Check sheet for the modelled part. Datum: model origin and axes. Units: mm. Face numbers are marked on the shaded views. A direction names the side the tool comes from. Round coordinates to 2 decimals unless told otherwise and drop trailing zeros. Order: outer loops, then holes, each group sorted by start corner. A loop starts at its lowest first (then second) coordinate and runs counter-clockwise, first axis right, second up. Notation, with made-up numbers: (-13, 39.5) -> (25, 39.5) arc R35 ccw to (25, 78.5) -> close; hole circle Ø3 at (-9.5, 52.25). An arc over 180 degrees is marked (long way). Answer as CSV lines item,"result". Start each with the question number.
from build123d import *

# Parameters (mm, degrees)
SKETCH1_W      = 16
SKETCH1_H      = 16
EXTRUDE1_DEPTH = 80
SKETCH2_W      = 13
SKETCH2_H      = 13
EXTRUDE2_DEPTH = 84.138438763
SKETCH3_R      = 4
SKETCH3_R_2    = 1.85
EXTRUDE3_DEPTH = 84.138438763
SKETCH4_R      = 4
SKETCH4_R_2    = 1.85
EXTRUDE4_DEPTH = 84.138438763
FILLET1_R      = 1


with BuildPart() as part:
    # Sketch1 → Extrude1 (new body)
    with BuildSketch(Plane.XY):
        with Locations((8, 8)):
            Rectangle(SKETCH1_W, SKETCH1_H)
    extrude(amount=-EXTRUDE1_DEPTH)

    # Sketch2 → Extrude2 (cut, through all)
    with BuildSketch(Plane.XY):
        with Locations((8, 8)):
            Rectangle(SKETCH2_W, SKETCH2_H)
    extrude(amount=-EXTRUDE2_DEPTH, mode=Mode.SUBTRACT)

    # Sketch3 → Extrude3 (cut, through all)
    with BuildSketch(Plane(origin=(0, 16, 0), x_dir=(1, 0, 0), z_dir=(0, 1, 0))):
        with Locations(Location((8, 64, 0), (0, 0, 270))):
            Circle(SKETCH3_R)
        with Locations(Location((8, 32, 0), (0, 0, 270))):
            Circle(SKETCH3_R)
        with Locations((8, 0)):
            Circle(SKETCH3_R)
        with Locations((8, 96)):
            Circle(SKETCH3_R)
        with Locations((8, 128)):
            Circle(SKETCH3_R)
        with Locations((8, 160)):
            Circle(SKETCH3_R)
        with Locations((8, 192)):
            Circle(SKETCH3_R)
        with Locations((8, 224)):
            Circle(SKETCH3_R)
        with Locations((8, 256)):
            Circle(SKETCH3_R)
        with Locations(Location((8, 48, 0), (0, 0, 270))):
            Circle(SKETCH3_R)
        with Locations(Location((8, 56, 0), (0, 0, 270))):
            Circle(SKETCH3_R_2)
        with Locations(Location((8, 40, 0), (0, 0, 270))):
            Circle(SKETCH3_R_2)
        with Locations((8, 80)):
            Circle(SKETCH3_R)
        with Locations((8, 88)):
            Circle(SKETCH3_R_2)
        with Locations(Location((8, 72, 0), (0, 0, 270))):
            Circle(SKETCH3_R_2)
        with Locations(Location((8, 16, 0), (0, 0, 270))):
            Circle(SKETCH3_R)
        with Locations(Location((8, 24, 0), (0, 0, 270))):
            Circle(SKETCH3_R_2)
        with Locations(Location((8, 8, 0), (0, 0, 270))):
            Circle(SKETCH3_R_2)
        with Locations((8, 112)):
            Circle(SKETCH3_R)
        with Locations((8, 120)):
            Circle(SKETCH3_R_2)
        with Locations((8, 104)):
            Circle(SKETCH3_R_2)
        with Locations((8, 144)):
            Circle(SKETCH3_R)
        with Locations((8, 152)):
            Circle(SKETCH3_R_2)
        with Locations((8, 136)):
            Circle(SKETCH3_R_2)
        with Locations((8, 176)):
            Circle(SKETCH3_R)
        with Locations((8, 184)):
            Circle(SKETCH3_R_2)
        with Locations((8, 168)):
            Circle(SKETCH3_R_2)
        with Locations((8, 208)):
            Circle(SKETCH3_R)
        with Locations((8, 216)):
            Circle(SKETCH3_R_2)
        with Locations((8, 200)):
            Circle(SKETCH3_R_2)
        with Locations((8, 240)):
            Circle(SKETCH3_R)
        with Locations((8, 248)):
            Circle(SKETCH3_R_2)
        with Locations((8, 232)):
            Circle(SKETCH3_R_2)
    extrude(amount=-EXTRUDE3_DEPTH, mode=Mode.SUBTRACT)

    # Sketch4 → Extrude4 (cut, through all)
    with BuildSketch(Plane(origin=(16, 0, 0), x_dir=(0, 0, -1), z_dir=(1, 0, 0))):
        with Locations(Location((32, 8, 0), (0, 0, 90))):
            Circle(SKETCH4_R)
        with Locations(Location((64, 8, 0), (0, 0, 90))):
            Circle(SKETCH4_R)
        with Locations((0, 8)):
            Circle(SKETCH4_R)
        with Locations((96, 8)):
            Circle(SKETCH4_R)
        with Locations((128, 8)):
            Circle(SKETCH4_R)
        with Locations((160, 8)):
            Circle(SKETCH4_R)
        with Locations((192, 8)):
            Circle(SKETCH4_R)
        with Locations((224, 8)):
            Circle(SKETCH4_R)
        with Locations((256, 8)):
            Circle(SKETCH4_R)
        with Locations(Location((48, 8.074203, 0), (0, 0, 90))):
            Circle(SKETCH4_R)
        with Locations(Location((40, 8.074203, 0), (0, 0, 90))):
            Circle(SKETCH4_R_2)
        with Locations(Location((56, 8.074203, 0), (0, 0, 90))):
            Circle(SKETCH4_R_2)
        with Locations((80, 8)):
            Circle(SKETCH4_R)
        with Locations(Location((72, 8, 0), (0, 0, 90))):
            Circle(SKETCH4_R_2)
        with Locations((88, 8)):
            Circle(SKETCH4_R_2)
        with Locations(Location((16, 8, 0), (0, 0, 90))):
            Circle(SKETCH4_R)
        with Locations(Location((8, 8, 0), (0, 0, 90))):
            Circle(SKETCH4_R_2)
        with Locations(Location((24, 8, 0), (0, 0, 90))):
            Circle(SKETCH4_R_2)
        with Locations((112, 8)):
            Circle(SKETCH4_R)
        with Locations((104, 8)):
            Circle(SKETCH4_R_2)
        with Locations((120, 8)):
            Circle(SKETCH4_R_2)
        with Locations((144, 8)):
            Circle(SKETCH4_R)
        with Locations((136, 8)):
            Circle(SKETCH4_R_2)
        with Locations((152, 8)):
            Circle(SKETCH4_R_2)
        with Locations((176, 8)):
            Circle(SKETCH4_R)
        with Locations((168, 8)):
            Circle(SKETCH4_R_2)
        with Locations((184, 8)):
            Circle(SKETCH4_R_2)
        with Locations((208, 8)):
            Circle(SKETCH4_R)
        with Locations((200, 8)):
            Circle(SKETCH4_R_2)
        with Locations((216, 8)):
            Circle(SKETCH4_R_2)
        with Locations((240, 8)):
            Circle(SKETCH4_R)
        with Locations((232, 8)):
            Circle(SKETCH4_R_2)
        with Locations((248, 8)):
            Circle(SKETCH4_R_2)
    extrude(amount=-EXTRUDE4_DEPTH, mode=Mode.SUBTRACT)

    # Fillet1
    fillet1_edges = [part.edges().sort_by_distance(p)[0] for p in [
        (0, 16, -40),
        (16, 16, -40),
        (16, 0, -40),
        (0, 0, -40),
    ]]
    fillet(fillet1_edges, radius=FILLET1_R)


solid = part.part
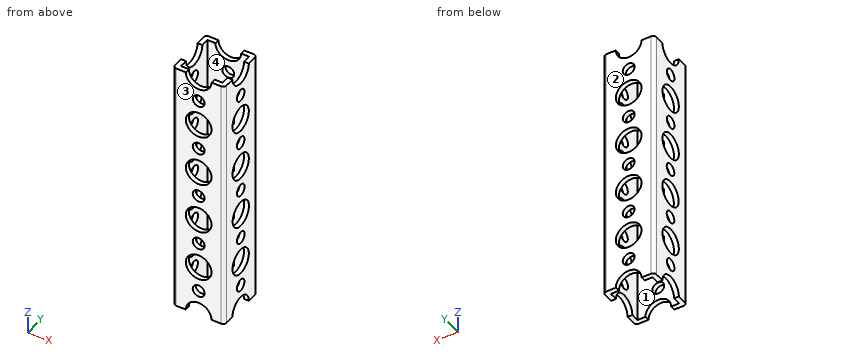
1) Section check B-B on x = 13. Record the cut outline in (y, z), then the cut area to 3 significant figures.
2) Depth check by flat-ended pin: pin 1 Ø6 at (y, z) = (8, -8) entering from +X. Enter the tip coordinate at first touch or a pass-through.
3) Access from +Z, -Z, +X, -X, +Y, -Y to the whole of each face (thin tool, end or side, straight path). Record for the marked faces 3 and 4.
4) Section check D-D on y = 8. Count the separate pieces of the cut face and the enclosed holes in it, then the cut area to 3 significant figures.
5) Mould release check, pull along X, two halves, no side actions. Record for the marked faces 1 and 2: released by +X, released by -X, zero draft, split by the parting line, or undercut.
6) Section check A-A on z = -72. Record the cut outline in (x, y), then the cut area to 3 significant figures.
7) Material ranges on line 1 along X through (y, z) = (13.5, -61.5); line 2 along X through (y, z) = (14.9, -32), recorded low to high.
8) Section check C-C on z = -16. Record the cut outline in (x, y), then the cut area to 3 significant figures.
Solutions:
1,outline,"(0, -80) -> (1.5, -80) -> (1.5, 0) -> (0, 0) -> close; (14.5, -80) -> (16, -80) -> (16, 0) -> (14.5, 0) -> close"
1,area,"240 mm^2"
2,pin 1,"stops at x = 16"
3,face 3,"+Z, -Z, +X, -X, -Y"
3,face 4,"+Z, -Z"
4,separate pieces,"20"
4,enclosed holes,"0"
4,area,"64.5 mm^2"
5,face 1,"undercut"
5,face 2,"zero draft"
6,outline,"(0, 1) arc R1 ccw to (1, 0) -> (6.15, 0) -> (6.15, 1.5) -> (1.5, 1.5) -> (1.5, 6.15) -> (0, 6.15) -> close; (0, 9.85) -> (1.5, 9.85) -> (1.5, 14.5) -> (6.15, 14.5) -> (6.15, 16) -> (1, 16) arc R1 ccw to (0, 15) -> close; (9.85, 0) -> (15, 0) arc R1 ccw to (16, 1) -> (16, 6.15) -> (14.5, 6.15) -> (14.5, 1.5) -> (9.85, 1.5) -> close; (9.85, 14.5) -> (14.5, 14.5) -> (14.5, 9.85) -> (16, 9.85) -> (16, 15) arc R1 ccw to (15, 16) -> (9.85, 16) -> close"
6,area,"63.9 mm^2"
7,line 1,"x = 0 to 1.5, 14.5 to 16"
7,line 2,"x = 0 to 4, 12 to 16"
8,outline,"(0, 1) arc R1 ccw to (1, 0) -> (4, 0) -> (4, 1.5) -> (1.5, 1.5) -> (1.5, 4) -> (0, 4) -> close; (0, 12) -> (1.5, 12) -> (1.5, 14.5) -> (4, 14.5) -> (4, 16) -> (1, 16) arc R1 ccw to (0, 15) -> close; (12, 0) -> (15, 0) arc R1 ccw to (16, 1) -> (16, 4) -> (14.5, 4) -> (14.5, 1.5) -> (12, 1.5) -> close; (12, 14.5) -> (14.5, 14.5) -> (14.5, 12) -> (16, 12) -> (16, 15) arc R1 ccw to (15, 16) -> (12, 16) -> close"
8,area,"38.1 mm^2"
